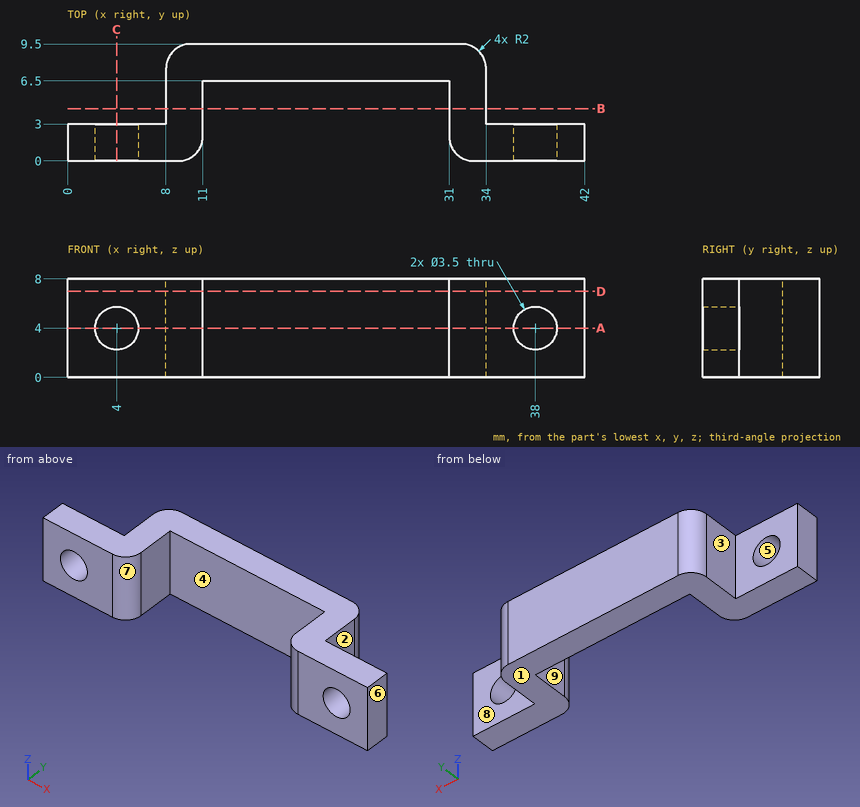
Check sheet for the drawn part. Datum: minimum x, y, z corner. Units: mm. A direction names the side the tool comes from. Coordinates: 2 decimals unless noted, no trailing zeros. Order: outer loops, then holes, each group sorted by start corner. A loop starts at its lowest first (then second) coordinate and runs counter-clockwise, first axis right, second up. Notation, with made-up numbers: M 31,-17.5 L 81,-17.5 A6 ccw 81,-8.5 Z; hole C 58,82 d1. An arc over 180 degrees is marked long. One line per item, written item: value. Start each with the question number.
Item 1: Sectioned sample at D-D (z = 7). Enter the section's corners in (x, y).
Item 2: Scan lines: probe 1 along X at (y, z) = (2.3, 4); probe 2 along X at (y, z) = (1.1, 4); probe 3 along Z at (x, y) = (38, 0.6). Record each from-to range of solid material in increasing order.
Item 3: Mould release check, pull along X, two halves, no side actions. Record for the marked faces 6, 7, 8 and 9: released by +X, released by -X, zero draft, split by the parting line, or undercut.
Item 4: Sectioned sample at B-B (y = 4.25). Enter the section's corners in (x, z), then the cut area to 3 significant figures.
Item 5: Gauge pin test, flat ends, axial feed: pin 1 (1.3 mm diameter, centred on y = 5, z = 4, fed in from +X); pin 2 (1.3 mm diameter, centred on y = 5, z = 3.5, fed in from -X); pin 3 (1.3 mm diameter, centred on y = 3.5, z = 4, fed in from +X); pin 4 (2.5 mm diameter, centred on x = 37.5, z = 3.5, fed in from +Y). Record the tip position at first contact, or that the pin passes through.
Item 6: Sectioned sample at A-A (z = 4). Enter the section's corners in (x, y), then the cut area to 3 significant figures.
Item 7: Access from +Z, -Z, +X, -X, +Y, -Y to the whole of each face (thin tool, end or side, straight path). Record for the marked faces 1, 2, 3, 4 and 5.
Item 8: Sectioned sample at C-C (x = 4). Enter the section's corners in (y, z), then the cut area to 3 significant figures.
Conclusion:
1. outline: M 0,0 L 9,0 A2 ccw 11,2 L 11,6.5 L 31,6.5 L 31,2 A2 ccw 33,0 L 42,0 L 42,3 L 34,3 L 34,7.5 A2 ccw 32,9.5 L 10,9.5 A2 ccw 8,7.5 L 8,3 L 0,3 Z
2. probe 1: x = 0 to 2.25, 5.75 to 11, 31 to 36.25, 39.75 to 42
2. probe 2: x = 0 to 2.25, 5.75 to 10.79, 31.21 to 36.25, 39.75 to 42
2. probe 3: z = 0 to 2.25, 5.75 to 8
3. face 6: released by +X
3. face 7: undercut
3. face 8: zero draft
3. face 9: undercut
4. outline: M 8,0 L 11,0 L 11,8 L 8,8 Z; M 31,0 L 34,0 L 34,8 L 31,8 Z
4. area: 48.0 mm^2
5. pin 1: stops at x = 34
5. pin 2: stops at x = 8
5. pin 3: stops at x = 42
5. pin 4: stops at y = 3
6. outline: M 0,0 L 2.25,0 L 2.25,3 L 0,3 Z; M 5.75,0 L 9,0 A2 ccw 11,2 L 11,6.5 L 31,6.5 L 31,2 A2 ccw 33,0 L 36.25,0 L 36.25,3 L 34,3 L 34,7.5 A2 ccw 32,9.5 L 10,9.5 A2 ccw 8,7.5 L 8,3 L 5.75,3 Z; M 39.75,0 L 42,0 L 42,3 L 39.75,3 Z
6. area: 141 mm^2
7. face 1: -Z, +X, -X, +Y, -Y
7. face 2: +Z, -Z, +X, +Y
7. face 3: +Z, -Z, -X, +Y
7. face 4: +Z, -Z, -Y
7. face 5: +Y, -Y
8. outline: M 0,0 L 3,0 L 3,2.25 L 0,2.25 Z; M 0,5.75 L 3,5.75 L 3,8 L 0,8 Z
8. area: 13.5 mm^2
